Part model, mm, in its own coordinate system. A direction names the side the tool comes from. Round coordinates to 2 decimals unless told otherwise and drop trailing zeros. Write each loop counter-clockwise with the first axis right and the second up, starting at its lowest first coordinate (ties: lowest second). Pieces come first, ordered by that corner, then holes.
```python
from build123d import *

# Parameters (mm, degrees)
F0_W     = 10
F0_H     = 10
F1_DEPTH = 10
F2_R     = 4.99999
F3_R     = 10
F4_SIZE  = 2


# Not quite as in the source:
# - a fillet or chamfer is up to 0.001 mm smaller than in the source, because OpenCascade refuses the exact size


with BuildPart() as f1:
    # F0 (on Top) → F1 (new body)
    with BuildSketch(Plane.XY):
        Polygon((6.4705845391, 30), (6.4705845391, 40), (-23.5294154609, 40), (-23.5294154609, 30), (-13.5294154609, 30), align=None)
        Polygon((16.4705845391, 40), (6.4705845391, 40), (6.4705845391, 30), (6.4705845391, 20), (16.4705845391, 20), align=None)
        Polygon((-13.5294154609, -10), (-13.5294154609, 30), (-23.5294154609, 30), (-23.5294154609, -20), (-13.5294154609, -20), align=None)
        Polygon((6.4705845391, -10), (-13.5294154609, -10), (-13.5294154609, -20), (16.4705845391, -20), (16.4705845391, -10), align=None)
        with Locations((11.4705845391, -5)):
            Rectangle(F0_W, F0_H)
    extrude(amount=F1_DEPTH)

    # F2 (radius 5 in the source; OpenCascade refuses exactly that, so slightly less here)
    f2_edges = [f1.edges().sort_by_distance(p)[0] for p in [
        (16.470585, 0, 5),
        (6.470585, 0, 5),
        (-13.529415, -10, 5),
        (6.470585, -10, 5),
        (6.470585, 20, 5),
        (6.470585, 30, 5),
        (-13.529415, 30, 5),
        (16.470585, 20, 5),
    ]]
    fillet(f2_edges, radius=F2_R)

    # F3
    f3_edges = [f1.edges().sort_by_distance(p)[0] for p in [
        (16.470585, 40, 5),
        (-23.529415, 40, 5),
        (16.470585, -20, 5),
        (-23.529415, -20, 5),
    ]]
    fillet(f3_edges, radius=F3_R)

    # F4
    f4_edges = [f1.edges().sort_by_distance(p)[0] for p in [
        (16.470585, 27.499995, 10),
        (13.541652, 37.071068, 10),
        (15.006121, 21.464463, 10),
        (-3.529415, 40, 10),
        (11.470585, 20, 10),
        (-20.600483, 37.071068, 10),
        (7.935048, 21.464463, 10),
        (-23.529415, 10, 10),
        (6.470585, 25, 10),
        (-20.600483, -17.071068, 10),
        (5.006121, 28.535537, 10),
        (-3.529415, -20, 10),
        (-3.529415, 30, 10),
        (13.541652, -17.071068, 10),
        (-12.064952, 28.535537, 10),
        (16.470585, -7.499995, 10),
        (-13.529415, 10, 10),
        (15.006121, -1.464463, 10),
        (-12.064952, -8.535537, 10),
        (11.470585, 0, 10),
        (-3.529415, -10, 10),
        (7.935048, -1.464463, 10),
        (5.006121, -8.535537, 10),
        (6.470585, -5, 10),
        (16.470585, 27.499995, 0),
        (13.541652, 37.071068, 0),
        (15.006121, 21.464463, 0),
        (-3.529415, 40, 0),
        (11.470585, 20, 0),
        (-20.600483, 37.071068, 0),
        (7.935048, 21.464463, 0),
        (-23.529415, 10, 0),
        (6.470585, 25, 0),
        (-20.600483, -17.071068, 0),
        (5.006121, 28.535537, 0),
        (-3.529415, -20, 0),
        (-3.529415, 30, 0),
        (13.541652, -17.071068, 0),
        (-12.064952, 28.535537, 0),
        (16.470585, -7.499995, 0),
        (-13.529415, 10, 0),
        (15.006121, -1.464463, 0),
        (-12.064952, -8.535537, 0),
        (11.470585, 0, 0),
        (-3.529415, -10, 0),
        (7.935048, -1.464463, 0),
        (5.006121, -8.535537, 0),
        (6.470585, -5, 0),
    ]]
    chamfer(f4_edges, length=F4_SIZE)


solid = f1.part
```
Q1. Cut at A-A on x = -5.5. Write the cut outline in (y, z).
Values follow:
outline: (-20, 2) - (-18, 0) - (-12, 0) - (-10, 2) - (-10, 8) - (-12, 10) - (-18, 10) - (-20, 8) - close; (30, 2) - (32, 0) - (38, 0) - (40, 2) - (40, 8) - (38, 10) - (32, 10) - (30, 8) - close
Q2. Cut at B-B on y = 8.5. Write the cut outline in (x, z).
Values follow:
outline: (-23.53, 2) - (-21.53, 0) - (-15.53, 0) - (-13.53, 2) - (-13.53, 8) - (-15.53, 10) - (-21.53, 10) - (-23.53, 8) - close
Q3. Which spindle directions (+Z, -Z, +X, -X, +Y, -Y) get a long thin tool onto all of the face, cutting with end or side? Do faces 4 (the cylindrical face through (15.04, -1.5, 5.04)), 5 (the conical face through (14.18, -2.35, 0.79)), 6 (the flat face through (-14.52, 9.79, 8.99)), 7 (the conical face through (-13, 29, 1)). Say none if no direction does.
Values follow:
face 4: +Z, -Z, +X
face 5: -Z, +X
face 6: +Z
face 7: -Z
Q4. Wall check: L1, parallel to Y at x = -2.5, z = 4.25; L2, parallel to X at y = 15, z = 3.75; L3, parallel to X at y = 28.5, z = 7.5. Give the ranges that are in metal, low to high.
Values follow:
L1: y = -20 to -10, 30 to 40
L2: x = -23.53 to -13.53
L3: x = -23.53 to -12.1, 5.04 to 16.47
Q5. Mould opens along Y. For faces 1 (the cylindrical face through (8, -1.4, 5)), 2 (the conical face through (-19.66, -15.99, 9.43)), 3 (the flat face through (-22.54, 10.28, 8.99)) say: +Y half, -Y half, draft (parallel to the pull), parting line (faces both ways), or undercut.
Values follow:
face 1: undercut
face 2: -Y half
face 3: draft
Q6. Drop flat-ended pins along their axis: pin 1 (5 mm diameter, centred on x = -19.5, z = 7.5, fed in from +Y); pin 2 (2 mm diameter, centred on x = -14, y = 24, fed in from -Z); pin 3 (3 mm diameter, centred on y = 5.5, z = 4.5, fed in from +X); pin 4 (5 mm diameter, centred on y = 22.5, z = 5, fed in from +X). Give the stop position or say it passes through.
Values follow:
pin 1: stops at y = 39.38
pin 2: stops at z = 0.53
pin 3: stops at x = -13.53
pin 4: stops at x = 16.47
